Part model, mm, in its own coordinate system. Give positions to 0.01 mm unless a question says otherwise; leave off trailing zeros. Write each loop counter-clockwise with the first axis right and the second up, starting at its lowest first coordinate (ties: lowest second). Pieces come first, ordered by that corner, then holes. Notation, with made-up numbers: M 81,-14 L 88,-14 A9 cw 88,-7 Z; hole C 11,53.25 d11. An arc over 180 degrees is marked long. Answer as CSV lines item,"result". Start each with the question number.
1) Slice it at B-B, the plane x = 14.5. Give the cut face in (y, z), plus the area to 3 significant figures.
2) Wall check: line 1 along X through (y, z) = (13.5, 25); line 2 along X through (y, z) = (15.5, 41); line 3 along Y through (x, z) = (15, 30.5). Give the ranges that are in metal, low to high. Write a range as from..to.
3) Slice it at C-C, the plane x = 5. Give the cut face in (y, z).
4) Pin check, flat tips, straight feed: pin 1 Ø4.5 at (x, y) = (15, 15.5) entering from +Z; pin 2 Ø1.5 at (x, z) = (10.5, 14) entering from -Y. Stop position of each tip, or through.
5) Mould opens along X. For faces 1 (the cylindrical face through (16.03, 14.55, 35.53)), 2 (the flat face through (10, 15, 72.07)), 3 (the flat face through (20, 12, 36)) say: pulls with the +X half, pulls with the -X half, needs draft (parallel to the pull), parting line crosses it, or undercut.
6) Slice it at D-D, the plane y = 2. Give the cut face in (x, z), plus the area to 3 significant figures.
7) Slice it at A-A, the plane z = 43. Give the cut face in (x, y).
```python
from build123d import *

# Parameters (mm, degrees)
SKETCH1_R           = 1.4
BOSS_EXTRUDE1_DEPTH = 72.07


with BuildPart() as part:
    # Sketch1 → Boss-Extrude1 (new body)
    with BuildSketch(Plane.XY):
        with BuildLine():
            Line((0, 0), (1.01, 0))
            ThreePointArc((1.01, 0), (8.762779495, 9.744229061), (20, 4.379486271))
            Line((20, 4.379486271), (20, 20))
            Line((20, 20), (0, 20))
            Line((0, 20), (0, 0))
        make_face()
        with Locations(Location((5, 13.5, 0), (0, 0, 180))):
            Circle(SKETCH1_R, mode=Mode.SUBTRACT)
        with Locations(Location((15, 15.5, 0), (0, 0, 180))):
            Circle(SKETCH1_R, mode=Mode.SUBTRACT)
    extrude(amount=BOSS_EXTRUDE1_DEPTH)


solid = part.part
```
Found:
1,outline,"M 9.37,0 L 14.19,0 L 14.19,72.07 L 9.37,72.07 Z; M 16.81,0 L 20,0 L 20,72.07 L 16.81,72.07 Z"
1,area,"578 mm²"
2,line 1,"0..3.6, 6.4..20"
2,line 2,"0..13.6, 16.4..20"
2,line 3,"9.17..14.1, 16.9..20"
3,outline,"M 7.99,0 L 12.1,0 L 12.1,72.07 L 7.99,72.07 Z; M 14.9,0 L 20,0 L 20,72.07 L 14.9,72.07 Z"
4,pin 1,"z = 72.07"
4,pin 2,"y = 9.92"
5,face 1,"undercut"
5,face 2,"needs draft"
5,face 3,"pulls with the +X half"
6,outline,"M 0,0 L 1.21,0 L 1.21,72.07 L 0,72.07 Z"
6,area,"87.4 mm²"
7,outline,"M 0,0 L 1.01,0 A10 cw 20,4.38 L 20,20 L 0,20 Z; hole C 5,13.5 d2.8; hole C 15,15.5 d2.8"
